from build123d import *

# Parameters (mm, degrees)
F1_DEPTH = 19.05
F3_DEPTH = 19.051
F4_R     = 3.429
F5_DEPTH = 31.751
F6_W     = 11.176
F6_H     = 19.05
F7_DEPTH = 9.525
F8_R     = 3.429
F9_DEPTH = 31.751


with BuildPart() as f1:
    # F0 (on Top) → F1 (new body)
    with BuildSketch(Plane.XY):
        Polygon((-31.75, 19.05), (-31.75, 0), (31.75, 0), (31.75, 19.05), (16.51, 19.05), (16.51, 31.75), (-16.51, 31.75), (-16.51, 19.05), align=None)
    extrude(amount=F1_DEPTH)

    # F2 (on Top) → F3 (cut, through all)
    with BuildSketch(Plane.XY):
        with BuildLine():
            Line((-7.62, 18.415), (-4.848091, 18.415))
            ThreePointArc((-4.848091, 18.415), (0, 14.1605), (4.848091, 18.415))
            Line((4.848091, 18.415), (16.51, 18.415))
            Line((16.51, 18.415), (16.51, 19.685))
            Line((16.51, 19.685), (4.848091, 19.685))
            ThreePointArc((4.848091, 19.685), (0, 23.9395), (-4.848091, 19.685))
            Line((-4.848091, 19.685), (-7.62, 19.685))
            ThreePointArc((-7.62, 19.685), (-8.255, 19.05), (-7.62, 18.415))
        make_face()
    extrude(amount=F3_DEPTH, mode=Mode.SUBTRACT)

    # F4 (on Front) → F5 (cut, through all)
    with BuildSketch(Plane.XZ):
        with Locations((25.4, 9.525)):
            Circle(F4_R)
        with Locations((-25.4, 9.525)):
            Circle(F4_R)
    extrude(amount=-F5_DEPTH, mode=Mode.SUBTRACT)

    # F6 (on Front) → F7 (cut)
    with BuildSketch(Plane.XZ):
        with Locations((9.525, 9.525)):
            Rectangle(F6_W, F6_H)
    extrude(amount=-F7_DEPTH, mode=Mode.SUBTRACT)

    # F8 (on face) → F9 (cut, through all)
    with BuildSketch(Plane(origin=(0, 31.75, 0), x_dir=(-1, 0, 0), z_dir=(0, 1, 0))):
        with Locations((-9.525, 9.525)):
            Circle(F8_R)
    extrude(amount=-F9_DEPTH, mode=Mode.SUBTRACT)


solid = f1.part
Input: part model. Units: mm. Frame: model coordinates. A direction names the side the tool comes from. Coordinates: 2 decimals unless noted, no trailing zeros. Order: outer loops, then holes, each group sorted by start corner. A loop starts at its lowest first (then second) coordinate and runs counter-clockwise, first axis right, second up. Notation, with made-up numbers: M 53,83.5 L 91,83.5 A17 cw 91,116.5 Z; hole C 72.25,62 d9. An arc over 180 degrees is marked long. Answer in a Markdown table with one row per item.
(1) Section query A-A, the plane y = 11. Output: boundary loops of the cut face in (x, z) (3 decimals).
Numbers:
| item | result |
|---|---|
| outline | M -31.75,0 L 31.75,0 L 31.75,19.05 L -31.75,19.05 Z; hole C -25.4,9.525 d6.858; hole C 9.525,9.525 d6.858; hole C 25.4,9.525 d6.858 |
(2) Contact query for flat-ended pins moving along their axis: pin 1 Ø2 at (x, z) = (19, 16) entering from +Y; pin 2 Ø9.5 at (y, z) = (28, 12) entering from +X; pin 3 Ø8 at (x, z) = (9.525, 9.525) entering from -Y (3 decimals); pin 4 Ø6 at (x, z) = (9.525, 9.525) entering from +Y. Output: stop coordinate, or through.
Numbers:
| item | result |
|---|---|
| pin 1 | stops at y = 19.05 |
| pin 2 | stops at x = 16.51 |
| pin 3 | stops at y = 9.525 |
| pin 4 | passes through |
(3) Section query C-C, the plane y = 21. Output: boundary loops of the cut face in (x, z) (3 decimals), plus the area to 3 significant figures.
Numbers:
| item | result |
|---|---|
| outline | M -16.51,0 L -4.484,0 L -4.484,19.05 L -16.51,19.05 Z; M 4.484,0 L 16.51,0 L 16.51,19.05 L 4.484,19.05 Z; hole C 9.525,9.525 d6.858 |
| area | 421 mm^2 |
(4) Section query B-B, the plane x = 25.4. Output: boundary loops of the cut face in (y, z), plus the area to 3 significant figures.
Numbers:
| item | result |
|---|---|
| outline | M 0,0 L 19.05,0 L 19.05,6.1 L 0,6.1 Z; M 0,12.95 L 19.05,12.95 L 19.05,19.05 L 0,19.05 Z |
| area | 232 mm^2 |
(5) Material intervals for line 1 (X direction, y = 7, z = 9.5); line 2 (Y direction, x = 8.5, z = 13) (3 decimals); line 3 (X direction, y = 17, z = 9.75), sorted ascending. Write a range as [from, to].
Numbers:
| item | result |
|---|---|
| line 1 | x = [-31.75, -28.83], [-21.97, 3.94], [15.11, 21.97], [28.83, 31.75] |
| line 2 | y = [9.525, 18.415], [19.685, 31.75] |
| line 3 | x = [-31.75, -28.82], [-21.98, -4.44], [4.44, 6.1], [12.95, 21.98], [28.82, 31.75] |
(6) Access query for faces 1 (the flat face through (16.51, 26, 9)), 2 (the flat face through (5.7, 9.525, 9.7)), 3 (the cylindrical face through (0.1, 23.94, 9.39)), 4 (the flat face through (-16.51, 25, 9)). Directions: +Z, -Z, +X, -X, +Y, -Y. A direction counts if a zero-diameter tool reaches every point of the face in a straight line with its end or side. Return the directions, or none.
Numbers:
| item | result |
|---|---|
| face 1 | +Z, -Z, +X, +Y |
| face 2 | +Z, -Z, -Y |
| face 3 | +Z, -Z |
| face 4 | +Z, -Z, -X, +Y |
(7) Draft query along Y for faces 5 (the flat face through (-22, 19.05, 12)), 6 (the flat face through (-31.75, 10, 9)), 7 (the flat face through (-6, 18.415, 9)), 8 (the flat face through (21, 0, 9)). Return one class per face: pulls with the +Y half, pulls with the -Y half, needs draft (parallel to the pull), parting line crosses it, or undercut.
Numbers:
| item | result |
|---|---|
| face 5 | pulls with the +Y half |
| face 6 | needs draft |
| face 7 | undercut |
| face 8 | pulls with the -Y half |
